```python
from build123d import *

# Parameters (mm, degrees)
SKETCH1_W           = 15
SKETCH1_H           = 15
BOSS_EXTRUDE2_DEPTH = 4
SKETCH4_R           = 6
CUT_EXTRUDE4_DEPTH  = 3
SKETCH5_R           = 1.25
BOSS_EXTRUDE3_DEPTH = 2
FILLET2_R           = 1
SKETCH6_R           = 1
BOSS_EXTRUDE4_DEPTH = 1


with BuildPart() as part:
    # Sketch1 → Boss-Extrude2 (new body)
    with BuildSketch(Plane(origin=(0, 0, 0), x_dir=(1, 0, 0), z_dir=(0, 1, 0))):
        Rectangle(SKETCH1_W, SKETCH1_H)
    extrude(amount=BOSS_EXTRUDE2_DEPTH)

    # Sketch4 → Cut-Extrude4 (cut)
    with BuildSketch(Plane(origin=(0, 4, 0), x_dir=(1, 0, 0), z_dir=(0, 1, 0))):
        Circle(SKETCH4_R)
    extrude(amount=-CUT_EXTRUDE4_DEPTH, mode=Mode.SUBTRACT)

    # Sketch5 → Boss-Extrude3 (add)
    with BuildSketch(Plane(origin=(0, 1, 0), x_dir=(1, 0, 0), z_dir=(0, 1, 0))):
        Circle(SKETCH5_R)
    extrude(amount=BOSS_EXTRUDE3_DEPTH)

    # Fillet2
    fillet2_edges = [part.edges().sort_by_distance(p)[0] for p in [
        (-1.25, 3, 0),
    ]]
    fillet(fillet2_edges, radius=FILLET2_R)

    # Sketch6 → Boss-Extrude4 (add)
    with BuildSketch(Plane(origin=(0, 4, 0), x_dir=(1, 0, 0), z_dir=(0, 1, 0))):
        with Locations((-5.5, 5.5)):
            Circle(SKETCH6_R)
        with Locations((5.5, 5.5)):
            Circle(SKETCH6_R)
        with Locations((-5.5, -5.5)):
            Circle(SKETCH6_R)
        with Locations((5.5, -5.5)):
            Circle(SKETCH6_R)
    extrude(amount=BOSS_EXTRUDE4_DEPTH)


solid = part.part
```
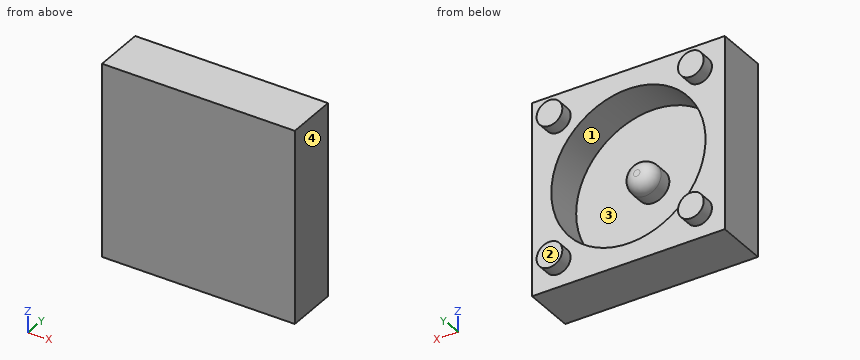
For this review, take the finished solid that the model builds, in its own axes (mm). Face numbers are marked on the shaded views. Give positions to 0.01 mm unless a question says otherwise; leave off trailing zeros. Order: outer loops, then holes, each group sorted by start corner. A loop starts at its lowest first (then second) coordinate and runs counter-clockwise, first axis right, second up.
1) Take a section at D-D (z = -5.25). Give the boundary of the cut face in (x, y), then the cut area to 3 significant figures.
2) Insertion check: pin 1 (6 mm diameter, centred on x = -2, z = 0, fed in from +Y). The pin has a flat end and moves straight along its axis. Give the tip position at first contact, or say it passes through.
3) Take a section at C-C (x = 5.5). Give the boundary of the cut face in (y, z).
4) The part is to be moulded in two halves that separate along X. For the marked faces 1, 2, 3 and 4, say which applies: released by +X, released by -X, zero draft, split by the parting line, or undercut.
5) Take a section at B-B (z = 3). Give the boundary of the cut face in (x, y), then the cut area to 3 significant figures.
6) Wall thickness on line 1 (X direction, y = 1.8, z = 0); line 2 (X direction, y = 1.85, z = 0.5): over which ranges is each line inside the solid? List them lowest first.
7) Take a section at A-A (x = -4). Give the boundary of the cut face in (y, z), then the cut area to 3 significant figures.
Derived:
1. outline: (-7.5, 0) - (7.5, 0) - (7.5, 4) - (6.47, 4) - (6.47, 5) - (4.53, 5) - (4.53, 4) - (2.9, 4) - (2.9, 1) - (-2.9, 1) - (-2.9, 4) - (-4.53, 4) - (-4.53, 5) - (-6.47, 5) - (-6.47, 4) - (-7.5, 4) - close
1. area: 46.4 mm2
2. pin 1: stops at y = 3
3. outline: (0, -7.5) - (4, -7.5) - (4, -6.5) - (5, -6.5) - (5, -4.5) - (4, -4.5) - (4, -2.4) - (1, -2.4) - (1, 2.4) - (4, 2.4) - (4, 4.5) - (5, 4.5) - (5, 6.5) - (4, 6.5) - (4, 7.5) - (0, 7.5) - close
4. face 1: undercut
4. face 2: zero draft
4. face 3: undercut
4. face 4: released by +X
5. outline: (-7.5, 0) - (7.5, 0) - (7.5, 4) - (5.2, 4) - (5.2, 1) - (-5.2, 1) - (-5.2, 4) - (-7.5, 4) - close
5. area: 28.8 mm2
6. line 1: x = -7.5 to -6, -1.25 to 1.25, 6 to 7.5
6. line 2: x = -7.5 to -5.98, -1.15 to 1.15, 5.98 to 7.5
7. outline: (0, -7.5) - (4, -7.5) - (4, -4.47) - (1, -4.47) - (1, 4.47) - (4, 4.47) - (4, 7.5) - (0, 7.5) - close
7. area: 33.2 mm2
